Geometry: final body of the model. Coordinates: model frame, mm. Face numbers are marked on the shaded views. A direction names the side the tool comes from. Round coordinates to 2 decimals unless told otherwise and drop trailing zeros. Loops run counter-clockwise (first coordinate to the right, second up) from the corner with the lowest first, then second, coordinate; pieces in that order, holes last. Notation, with made-up numbers: M -34.75,-26.5 L -17.75,-26.5 A24 ccw -17.75,12.5 Z; hole C 22.5,-33 d5. An arc over 180 degrees is marked long. Answer as a JSON object with one key per item and string values.
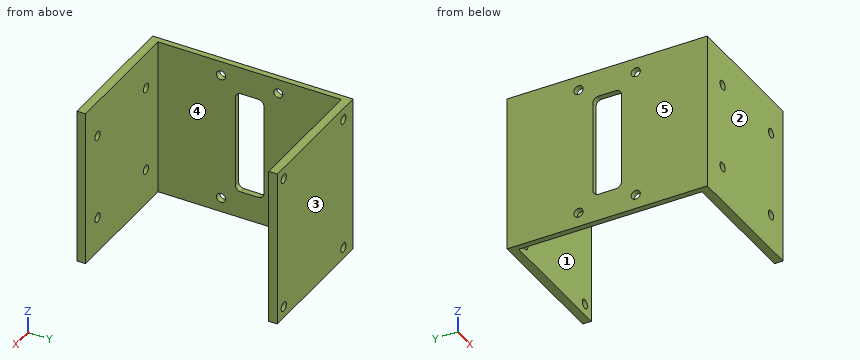
Autodesk Inventor part; units mm, degrees
ref_plane "YZ Plane" through (0, 0, 0) normal (1, 0, 0) x (0, 1, 0)
ref_plane "XZ Plane" through (0, 0, 0) normal (0, 1, 0) x (-1, 0, 0)
ref_plane "XY Plane" through (0, 0, 0) normal (0, 0, 1) x (1, 0, 0)
sketch "Skizze2" plane through (0, 0, 0) normal (1, 0, 0) x (0, 1, 0)
  line L0 (-49, 0) -> (49, 0)
  line L1 (0, -38.5) -> (0, 38.5)
  line L2 (35, 27.5) -> (-35, 27.5)
  line L3 (-35, 27.5) -> (-35, -27.5)
  line L4 (-35, -27.5) -> (35, -27.5)
  line L5 (35, -27.5) -> (35, 27.5)
  dimension "d5" = 70
  dimension "d6" = 55
extrude "Extrusion1" add sketch "Skizze2" along normal blind 2
sketch "Skizze3" plane through (2, 0, 0) normal (1, 0, 0) x (0, 0, -1)
  line L0 (-27.5, 35) -> (-27.5, -35)
  line L1 (27.5, -35) -> (27.5, 35)
  line L2 (-27.5, -35) -> (27.5, -35)
  line L3 (27.5, -35) -> (27.5, -32)
  line L4 (27.5, -32) -> (-27.5, -32)
  line L5 (-27.5, -32) -> (-27.5, -35)
  line L6 (27.5, 35) -> (-27.5, 35)
  line L7 (-27.5, 35) -> (27.5, 35)
  line L8 (27.5, 35) -> (27.5, 32)
  line L9 (27.5, 32) -> (-27.5, 32)
  line L10 (-27.5, 32) -> (-27.5, 35)
  point P0 (0, 0)
  point P1 (-27.5, -32)
  point P2 (-27.5, 32)
  point P3 (27.5, 32)
  dimension "d9" = 3
  dimension "d10" = 3
extrude "Extrusion2" add sketch "Skizze3" along normal blind 45 contours L6 L1 L9 L0 | L4 L1 L2 L0
sketch "Skizze5" plane through (0, 35, 27.5) normal (0, 1, 0) x (1, 0, 0)
  line L0 (0, 55) -> (0, 0)
  line L1 (0, 0) -> (47, 0)
  line L2 (0, 55) -> (47, 55)
  line L3 (47, 55) -> (47, 0)
  circle A0 centre (6, 4) radius 1.6
  circle A1 centre (6, 51) radius 1.6
  circle A2 centre (43, 51) radius 1.6
  circle A3 centre (43, 4) radius 1.6
  line L4 (56.4, 27.5) -> (-9.4, 27.5)
  point P0 (0, 27.5)
  dimension "d38" = 3.2
  dimension "d41" = 3.2
  dimension "d44" = 3.2
  dimension "d47" = 3.2
  dimension "d69" = 6
  dimension "d70" = 4
  dimension "d71" = 4
  dimension "d72" = 6
  dimension "d73" = 4
  dimension "d74" = 4
  dimension "d75" = 4
  dimension "d76" = 4
extrude "Extrusion3" cut sketch "Skizze5" against normal up to surface (3 mm away) contours A0 | A1 | A2 | A3
sketch "Skizze6" plane through (0, -35, -27.5) normal (0, -1, 0) x (1, 0, 0)
  circle A0 centre (39.5, 42.5) radius 1.6
  circle A1 centre (39.5, 12.5) radius 1.6
  circle A2 centre (9.5, 42.5) radius 1.6
  circle A3 centre (9.5, 12.5) radius 1.6
  line L0 (-9.4, 27.5) -> (56.4, 27.5)
  line L1 (0, 66) -> (0, -11)
  line L2 (47, 55) -> (47, 0)
  dimension "d52" = 3.2
  dimension "d53" = 3.2
  dimension "d63" = 3.2
  dimension "d65" = 3.2
  dimension "d84" = 15
  dimension "d86" = 9.5
  dimension "d87" = 9.5
  dimension "d88" = 15
  dimension "d89" = 15
  dimension "d90" = 7.5
  dimension "d91" = 7.5
  dimension "d92" = 15
extrude "Extrusion4" cut sketch "Skizze6" against normal up to surface (3 mm away)
sketch "Skizze7" plane through (0, 0, 0) normal (-1, 0, 0) x (0, 0, 1)
  circle A0 centre (22.5, -10) radius 1.6
  line L0 (27.5, -35) -> (-27.5, -35)
  line L1 (27.5, 35) -> (27.5, -35)
  circle A1 centre (-22.5, -10) radius 1.6
  line L2 (-27.5, -35) -> (-27.5, 35)
  circle A2 centre (22.5, 10) radius 1.6
  circle A3 centre (-22.5, 10) radius 1.6
  line L3 (18, -5) -> (-18, -5)
  line L4 (-18, -5) -> (-18, 5)
  line L5 (-18, 5) -> (18, 5)
  line L6 (18, 5) -> (18, -5)
  line L7 (-38.5, 0) -> (38.5, 0)
  line L8 (0, 49) -> (0, -49)
  point P0 (0, 0)
  dimension "d93" = 3.2
  dimension "d95" = 5
  dimension "d96" = 3.2
  dimension "d97" = 5
  dimension "d99" = 3.2
  dimension "d100" = 5
  dimension "d101" = 20
  dimension "d102" = 3.2
  dimension "d103" = 5
  dimension "d104" = 20
  dimension "d107" = 36
  dimension "d108" = 10
  dimension "d111" = 10
  dimension "d112" = 10
extrude "Extrusion5" cut sketch "Skizze7" against normal up to surface (2 mm away) contours A0 | A1 | A2 | A3
extrude "Extrusion6" cut sketch "Skizze7" against normal up to surface (2 mm away) contours L8 L7 L6 L3 | L3 L4 L7 L8 | L7 L8 L5 L6 | L7 L4 L5 L8
fillet "Rundung1" radius 2 4 edges at (1, 5, 18) (1, -5, 18) (1, -5, -18) (1, 5, -18)
properties part number "_3D-Druck"
1) First-contact query: pin 1 (3 mm diameter, centred on x = 6, z = 23.5, fed in from +Y); pin 2 (1.5 mm diameter, centred on y = 18.5, z = -5, fed in from +X); pin 3 (3.5 mm diameter, centred on x = 39.5, z = -15, fed in from -Y); pin 4 (3 mm diameter, centred on y = 10, z = 22.5, fed in from +X) (3 decimals). Flat tips, straight axial feed; report the tip coordinate or a pass-through.
Geometry results:
{"pin 1": "y = -32", "pin 2": "x = 2", "pin 3": "y = -35", "pin 4": "through"}
2) Cut plane C-C on y = 10. Return the cut outline in (x, z).
Geometry results:
{"outline": "M 0,-27.5 L 2,-27.5 L 2,-24.1 L 0,-24.1 Z; M 0,-20.9 L 2,-20.9 L 2,20.9 L 0,20.9 Z; M 0,24.1 L 2,24.1 L 2,27.5 L 0,27.5 Z"}
3) Line query: probe 1 along Y at (x, z) = (0.8, 22.5); probe 2 along X at (y, z) = (33.55, 23.5); probe 3 along Z at (x, y) = (6, 33). Output: solid intervals per line, ascending.
Geometry results:
{"probe 1": "-35 to -11.6, -8.4 to 8.4, 11.6 to 35", "probe 2": "0 to 4.4, 7.6 to 41.4, 44.6 to 47", "probe 3": "-27.5 to -25.1, -21.9 to 21.9, 25.1 to 27.5"}
4) Set-up query: the marked faces 4 and 5. Return all of +Z, -Z, +X, -X, +Y, -Y with unobstructed straight access to the full face (end or side cutting, diameter ignored); none if empty.
Geometry results:
{"face 4": "+Z, -Z, +X", "face 5": "+Z, -Z, -X, +Y, -Y"}
5) Cut plane A-A on x = 19. Return the cut outline in (y, z), and give its area (3 significant figures).
Geometry results:
{"outline": "M -35,-27.5 L -32,-27.5 L -32,27.5 L -35,27.5 Z; M 32,-27.5 L 35,-27.5 L 35,27.5 L 32,27.5 Z", "area": "330 mm2"}
6) Pull-direction query (Y, two-part tool) for the marked faces 1, 2 and 3; classes: +Y half, -Y half, draft (parallel to the pull), parting line (faces both ways), or undercut.
Geometry results:
{"face 1": "undercut", "face 2": "-Y half", "face 3": "+Y half"}
7) Cut plane D-D on z = 15. Return the cut outline in (x, y).
Geometry results:
{"outline": "M 0,-35 L 7.9,-35 L 7.9,-32 L 2,-32 L 2,-5 L 0,-5 Z; M 0,5 L 2,5 L 2,32 L 47,32 L 47,35 L 0,35 Z; M 11.1,-35 L 37.9,-35 L 37.9,-32 L 11.1,-32 Z; M 41.1,-35 L 47,-35 L 47,-32 L 41.1,-32 Z"}
8) Cut plane B-B on z = -5. Return the cut outline in (x, y), and give its area (3 significant figures).
Geometry results:
{"outline": "M 0,-35 L 47,-35 L 47,-32 L 2,-32 L 2,-5 L 0,-5 Z; M 0,5 L 2,5 L 2,32 L 47,32 L 47,35 L 0,35 Z", "area": "390 mm2"}
